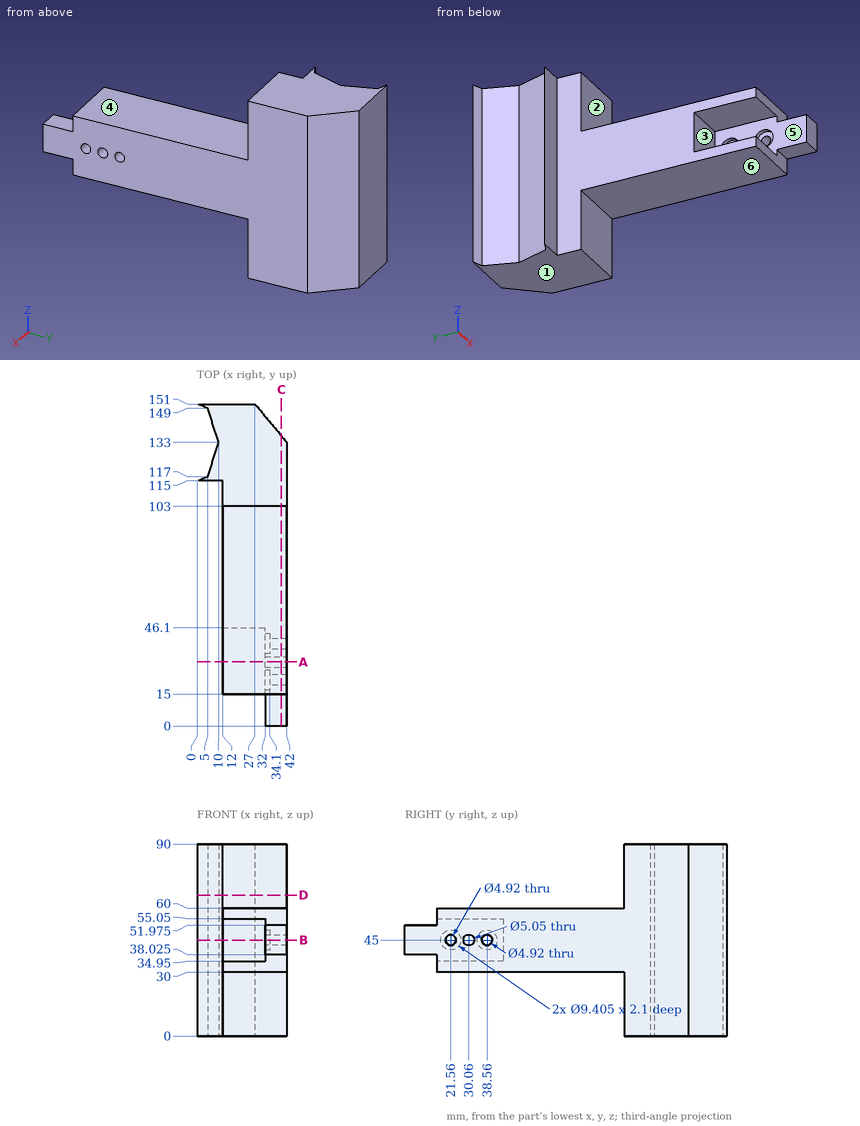
Here's the drawing with two shaded views (mm, measured from the low corner). I have some questions. A direction names the side the tool comes from. Coordinates: 2 decimals unless noted, no trailing zeros. Write each loop counter-clockwise with the first axis right and the second up, starting at its lowest first coordinate (ties: lowest second). Pieces come first, ordered by that corner, then holes. Notation, with made-up numbers: M 34.5,55 L 45.5,55 A25 ccw 45.5,92 Z; hole C 35.5,51.5 d10. An arc over 180 degrees is marked long. Answer as CSV lines item,"result".
Item 1: On a 3-axis mill with a long thin cutter (end or side, diameter ignored), from which of +Z, -Z, +X, -X, +Y, -Y can I reach the whole of each face in a straight line? I mean the marked faces 4, 5 and 6. Say none if no direction works.
Geometry results:
face 4,"+Z, +X, -X, -Y"
face 5,"-X, -Y"
face 6,"-Z, +X, -X, -Y"
Item 2: Please list where these lines run through material, in increasing order: line 1 along Y through (x, z) = (37, 45) (3 decimals); line 2 along Y through (x, z) = (36.25, 45) (3 decimals); line 3 along X through (y, z) = (102.5, 56).
Geometry results:
line 1,"y = 0 to 19.1, 24.02 to 27.535, 32.585 to 36.1, 41.02 to 139"
line 2,"y = 0 to 19.1, 24.02 to 27.535, 32.585 to 36.1, 41.02 to 139.9"
line 3,"x = 12 to 42"
Item 3: Imagine slicing it at C-C on x = 39.5. List the corners of the cut face in (y, z) for me (3 decimals), plus the area to 3 significant figures.
Geometry results:
outline,"M 0,38.025 L 15,38.025 L 15,30 L 103,30 L 103,0 L 136,0 L 136,90 L 103,90 L 103,60 L 15,60 L 15,51.975 L 0,51.975 Z; hole C 21.56,45 d4.92; hole C 30.06,45 d5.05; hole C 38.56,45 d4.92"
area,"5,760 mm2"
Item 4: I'm going to push flat-ended pins straight in: P1, Ø2, axis at x = 16, y = 54, coming from the -Z side; P2, Ø3, axis at x = 36.5, y = 5.5, coming from the +Z side (3 decimals); P3, Ø5.5, axis at y = 38.56, z = 45, coming from the -X side; P4, Ø8, axis at y = 30.06, z = 45, coming from the +X side. Where does each tip first touch, or does it pass through?
Geometry results:
P1,"stops at z = 30"
P2,"stops at z = 51.975"
P3,"stops at x = 34.1"
P4,"stops at x = 42"
Item 5: We'd pull the mould along Z, two halves only. Please class the marked faces 1, 2 and 3: +Z half, -Z half, draft (parallel to the pull), parting line (faces both ways), or undercut.
Geometry results:
face 1,"-Z half"
face 2,"draft"
face 3,"undercut"
Item 6: Imagine slicing it at D-D on z = 66. List the corners of the cut face in (x, y) for me.
Geometry results:
outline,"M 0,115 L 12,115 L 12,103 L 42,103 L 42,133 L 27,151 L 0,151 L 5,149 L 10,133 L 5,117 Z"
Item 7: Imagine slicing it at B-B on z = 45. State how many separate pieces and enclosed holes the cut face has, plus the area to 3 significant figures.
Geometry results:
separate pieces,"4"
enclosed holes,"0"
area,"3,490 mm2"
Item 8: Imagine slicing it at A-A on y = 30.06. List the corners of the cut face in (x, z) for me (3 decimals), plus the area to 4 significant figures.
Geometry results:
outline,"M 12,30 L 42,30 L 42,42.475 L 32,42.475 L 32,34.95 L 12,34.95 Z; M 12,55.05 L 32,55.05 L 32,47.525 L 42,47.525 L 42,60 L 12,60 Z"
area,"447.5 mm2"
